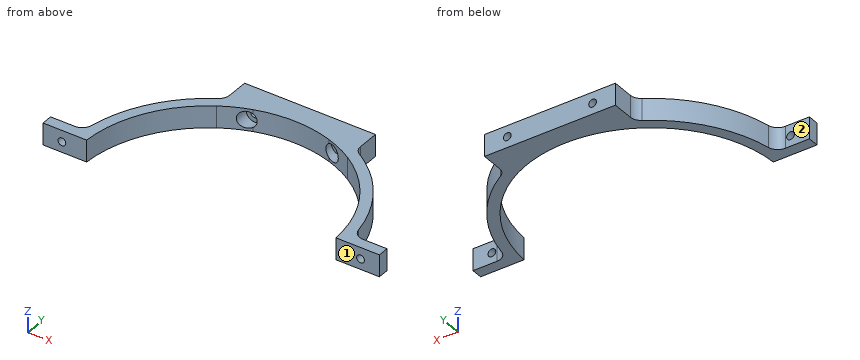
from build123d import *
from build123d import SkipClean  # not in build123d's __all__

# Parameters (mm, degrees)
F1_DEPTH       = 10
F3_D           = 3.556
F3_CBORE_D     = 7.62
F3_CBORE_DEPTH = 10
F4_DEPTH       = 10.0010001
F6_D           = 3.556
F7_R           = 5


with BuildPart() as f1:
    # F0 (on Top) → F1 (new body)
    with BuildSketch(Plane.XY):
        with BuildLine():
            ThreePointArc((30, 48.6428052234), (49.4079280032, 28.7224502859), (57.1149936532, 2))
            Line((57.1149936532, 2), (57.1149936532, 7))
            Line((57.1149936532, 7), (61.7545342465, 7))
            ThreePointArc((61.7545342465, 7), (51.6442091706, 34.5759766187), (30, 54.4299779533))
            Line((30, 54.4299779533), (30, 48.6428052234))
        make_face()
        with BuildLine():
            ThreePointArc((17.4212513902, 54.4299779533), (23.8865362266, 51.9187431194), (30, 48.6428052234))
            Line((30, 48.6428052234), (30, 54.4299779533))
            Line((30, 54.4299779533), (17.4212513902, 54.4299779533))
        make_face()
        with BuildLine():
            ThreePointArc((-17.4212513902, 54.4299779533), (0, 57.15), (17.4212513902, 54.4299779533))
            Line((17.4212513902, 54.4299779533), (30, 54.4299779533))
            ThreePointArc((30, 54.4299779533), (15.4886954339, 60.1890589207), (7.62e-08, 62.15))
            ThreePointArc((7.62e-08, 62.15), (-15.4886953601, 60.1890589397), (-30, 54.4299779533))
            Line((-30, 54.4299779533), (-17.4212513902, 54.4299779533))
        make_face()
        with BuildLine():
            Line((-30, 54.4299779533), (-30, 48.6428052234))
            ThreePointArc((-30, 48.6428052234), (-23.8865362266, 51.9187431194), (-17.4212513902, 54.4299779533))
            Line((-17.4212513902, 54.4299779533), (-30, 54.4299779533))
        make_face()
        with BuildLine():
            ThreePointArc((-57.1149936532, 2), (-49.4079280032, 28.7224502859), (-30, 48.6428052234))
            Line((-30, 48.6428052234), (-30, 54.4299779533))
            ThreePointArc((-30, 54.4299779533), (-51.6442091706, 34.5759766187), (-61.7545342465, 7))
            Line((-61.7545342465, 7), (-57.1149936532, 7))
            Line((-57.1149936532, 7), (-57.1149936532, 2))
        make_face()
        with BuildLine():
            Line((-77.1149936532, 2), (-62.1178114553, 2))
            ThreePointArc((-62.1178114553, 2), (-61.9866074843, 4.5036643506), (-61.7545342465, 7))
            Line((-61.7545342465, 7), (-77.1149936532, 7))
            Line((-77.1149936532, 7), (-77.1149936532, 2))
        make_face()
        with BuildLine():
            Line((-62.1178114553, 2), (-57.1149936532, 2))
            Line((-57.1149936532, 2), (-57.1149936532, 7))
            Line((-57.1149936532, 7), (-61.7545342465, 7))
            ThreePointArc((-61.7545342465, 7), (-61.9866074843, 4.5036643506), (-62.1178114553, 2))
        make_face()
        with BuildLine():
            Line((57.1149936532, 7), (57.1149936532, 2))
            Line((57.1149936532, 2), (62.1178114553, 2))
            ThreePointArc((62.1178114553, 2), (61.9866074843, 4.5036643506), (61.7545342465, 7))
            Line((61.7545342465, 7), (57.1149936532, 7))
        make_face()
        with BuildLine():
            ThreePointArc((61.7545342465, 7), (61.9866074843, 4.5036643506), (62.1178114553, 2))
            Line((62.1178114553, 2), (77.1149936532, 2))
            Line((77.1149936532, 2), (77.1149936532, 7))
            Line((77.1149936532, 7), (61.7545342465, 7))
        make_face()
        with BuildLine():
            Line((-30, 62.15), (-30, 54.4299779533))
            ThreePointArc((-30, 54.4299779533), (-15.4886953601, 60.1890589397), (7.62e-08, 62.15))
            Line((7.62e-08, 62.15), (-30, 62.15))
        make_face()
        with BuildLine():
            ThreePointArc((7.62e-08, 62.15), (15.4886954339, 60.1890589207), (30, 54.4299779533))
            Line((30, 54.4299779533), (30, 62.15))
            Line((30, 62.15), (7.62e-08, 62.15))
        make_face()
        with BuildLine():
            Line((-30, 48.6428052234), (30, 48.6428052234))
            ThreePointArc((30, 48.6428052234), (23.8865362266, 51.9187431194), (17.4212513902, 54.4299779533))
            Line((17.4212513902, 54.4299779533), (-17.4212513902, 54.4299779533))
            ThreePointArc((-17.4212513902, 54.4299779533), (-23.8865362266, 51.9187431194), (-30, 48.6428052234))
        make_face()
        Polygon((-30, 62.15), (7.62e-08, 62.15), (30, 62.15), (30, 67.15), (-30, 67.15), align=None)
    extrude(amount=F1_DEPTH)

    # F3 (through all)
    with Locations(Plane.XZ.offset(-48.6428052234)):
        with Locations((-19.558, 4.9517820589), (19.558, 4.9517820589)):
            CounterBoreHole(F3_D / 2, F3_CBORE_D / 2, F3_CBORE_DEPTH)

    # F0 (on Top) → F4 (cut, through all)
    with BuildSketch(Plane.XY):
        with BuildLine():
            Line((-30, 48.6428052234), (30, 48.6428052234))
            ThreePointArc((30, 48.6428052234), (23.8865362266, 51.9187431194), (17.4212513902, 54.4299779533))
            Line((17.4212513902, 54.4299779533), (-17.4212513902, 54.4299779533))
            ThreePointArc((-17.4212513902, 54.4299779533), (-23.8865362266, 51.9187431194), (-30, 48.6428052234))
        make_face()
    with SkipClean():  # cleaning this boolean's faces spoils the solid; the shape is the same uncleaned
        extrude(amount=F4_DEPTH, mode=Mode.SUBTRACT)

    # F6 (through all)
    with Locations(Plane.XZ.offset(-2)):
        with Locations((-68.453, 4.78035165), (68.453, 4.78035165)):
            Hole(F6_D / 2)

    # F7
    f7_edges = [f1.edges().sort_by_distance(p)[0] for p in [
        (-61.754534, 7, 5),
        (61.754534, 7, 5),
        (30, 54.429978, 5),
        (-30, 54.429978, 5),
    ]]
    fillet(f7_edges, radius=F7_R)


solid = f1.part
Input: part model. Units: mm. Frame: model coordinates. Face numbers are marked on the shaded views. A direction names the side the tool comes from. Round coordinates to 2 decimals unless told otherwise and drop trailing zeros. Order: outer loops, then holes, each group sorted by start corner. A loop starts at its lowest first (then second) coordinate and runs counter-clockwise, first axis right, second up.
1. Material intervals for line 1 (Z direction, x = -20, y = 54); line 2 (X direction, y = 43, z = 8); line 3 (X direction, y = 23, z = 3), sorted ascending.
The answers:
line 1: z = 0 to 1.17, 8.74 to 10
line 2: x = -44.87 to -37.64, 37.64 to 44.87
line 3: x = -57.74 to -52.32, 52.32 to 57.74
2. Cut plane A-A, the plane y = 40.5. Output: boundary loops of the cut face in (x, z).
The answers:
outline: (-47.14, 0) - (-40.32, 0) - (-40.32, 10) - (-47.14, 10) - close; (40.32, 0) - (47.14, 0) - (47.14, 10) - (40.32, 10) - close
3. Cut plane C-C, the plane x = 47.5. Output: boundary loops of the cut face in (y, z).
The answers:
outline: (31.78, 0) - (40.08, 0) - (40.08, 10) - (31.78, 10) - close
4. Set-up query: the marked faces 1 and 2. Return all of +Z, -Z, +X, -X, +Y, -Y with unobstructed straight access to the full face (end or side cutting, diameter ignored); none if empty.
The answers:
face 1: +Z, -Z, +X, -X, -Y
face 2: +Z, -Z, -X, +Y
5. Cut plane B-B, the plane y = 29.5. Output: boundary loops of the cut face in (x, z).
The answers:
outline: (-54.7, 0) - (-48.95, 0) - (-48.95, 10) - (-54.7, 10) - close; (48.95, 0) - (54.7, 0) - (54.7, 10) - (48.95, 10) - close
6. Cut plane D-D, the plane x = -48.5. Output: boundary loops of the cut face in (y, z).
The answers:
outline: (30.23, 0) - (38.86, 0) - (38.86, 10) - (30.23, 10) - close
7. Pin query (flat end, axial travel): P1, Ø1.5, axis at y = 8.5, z = 3.5, coming from the +X side; P2, Ø5, axis at y = 61, z = 3.5, coming from the +X side; P3, Ø1.5, axis at x = -30.5, z = 6.5, coming from the +Y side; P4, Ø6, axis at x = -20.5, z = 3.5, coming from the -Y side. Return the tip coordinate at first contact, or that it passes through.
The answers:
P1: stops at x = 63.44
P2: stops at x = 30
P3: stops at y = 67.15
P4: stops at y = 52.09
